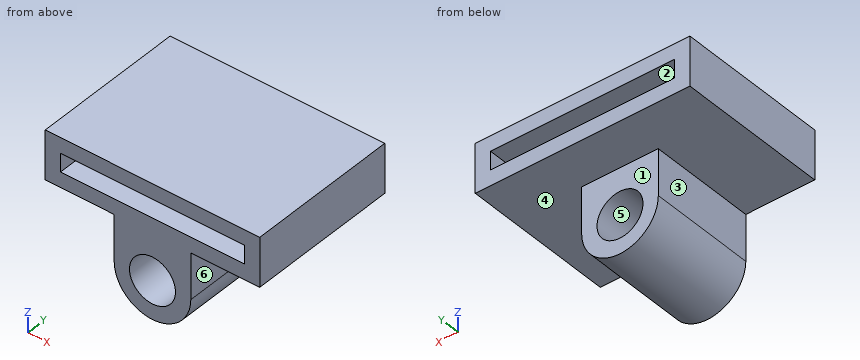
from build123d import *

# Parameters (mm, degrees)
SKETCH1_W                = 14
SKETCH1_H                = 3.2
SKETCH1_W_2              = 12
SKETCH1_H_2              = 1.2
BOSS_EXTRUDE1_DEPTH      = 5
BOSS_EXTRUDE2_DEPTH      = 2
BOSS_EXTRUDE2_DEPTH_BACK = 5
SKETCH1_3_R              = 1.5


with BuildPart() as part:
    # Sketch1 → Boss-Extrude1 (new, symmetric)
    with BuildSketch(Plane(origin=(0, 0, 0), x_dir=(1, 0, 0), z_dir=(0, 1, 0))):
        Rectangle(SKETCH1_W, SKETCH1_H)
        Rectangle(SKETCH1_W_2, SKETCH1_H_2, mode=Mode.SUBTRACT)
    extrude(amount=BOSS_EXTRUDE1_DEPTH, both=True)

    # Sketch1_3 → Boss-Extrude2 (add, two sides: drawn at the far end of the back side and taken through both)
    with BuildSketch(Plane(origin=(0, 0, 0), x_dir=(1, 0, 0), z_dir=(0, 1, 0)).offset(-BOSS_EXTRUDE2_DEPTH_BACK)):
        with BuildLine():
            ThreePointArc((2.5, 4.6), (0, 7.1), (-2.5, 4.6))
            Line((-2.5, 4.6), (-2.5, 1.6))
            Line((-2.5, 1.6), (2.5, 1.6))
            Line((2.5, 1.6), (2.5, 4.6))
        make_face()
        with Locations(Location((0, 4.6, 0), (0, 0, 270))):
            Circle(SKETCH1_3_R, mode=Mode.SUBTRACT)
    extrude(amount=BOSS_EXTRUDE2_DEPTH + BOSS_EXTRUDE2_DEPTH_BACK)


solid = part.part
Design review of the part built by this model. Coordinates are the model's own, in mm. Face numbers are marked on the shaded views. A direction names the side the tool comes from. Give positions to 0.01 mm unless a question says otherwise; leave off trailing zeros. Write each loop counter-clockwise with the first axis right and the second up, starting at its lowest first coordinate (ties: lowest second). Pieces come first, ordered by that corner, then holes. Notation, with made-up numbers: M 35.5,28.25 L 44.5,28.25 A24 cw 44.5,53.25 Z; hole C 36,-3 d7. An arc over 180 degrees is marked long. Return JSON: item names as keys, results as strings. Group by question number.
Item 1: Wall thickness on line 1 along X through (y, z) = (-3, -4.6); line 2 along Z through (x, y) = (4.5, -0.75); line 3 along X through (y, z) = (-4, 0.5): over which ranges is each line inside the solid? List them lowest first.
Item 2: Take a section at D-D (y = -3.75). Give the boundary of the cut face in (x, z).
Item 3: The part is to be moulded in two halves that separate along X. For the marked faces 4, 5 and 6, say which applies: pulls with the +X half, pulls with the -X half, needs draft (parallel to the pull), parting line crosses it, or undercut.
Item 4: Clearance check with flat-ended pins moving along their axes: pin 1 Ø2.5 at (y, z) = (-0.5, -3.5) entering from +X; pin 2 Ø1.5 at (x, z) = (5, -4.5) entering from +Y; pin 3 Ø3 at (x, z) = (4, -0.5) entering from -Y. State where each tip first meets the part, or that it passes through.
Item 5: Take a section at C-C (x = 5). Give the boundary of the cut face in (y, z), plus the area to 3 significant figures.
Item 6: Take a section at A-A (x = 0). Give the boundary of the cut face in (y, z), plus the area to 3 significant figures.
Item 7: Tool access review of the marked faces 1, 2 and 3: name each direction out of +Z, -Z, +X, -X, +Y, -Y from which nothing blocks a thin tool from reaching the whole face with its end or side.
Item 8: Take a section at B-B (y = 4.5). Give the boundary of the cut face in (x, z), plus the area to 3 significant figures.
Return value:
{
 "1": {"line 1": "x = -2.5 to -1.5, 1.5 to 2.5", "line 2": "z = -1.6 to -0.6, 0.6 to 1.6", "line 3": "x = -7 to -6, 6 to 7"},
 "2": {"outline": "M -7,-1.6 L -2.5,-1.6 L -2.5,-4.6 A2.5 ccw 2.5,-4.6 L 2.5,-1.6 L 7,-1.6 L 7,1.6 L -7,1.6 Z; hole M -6,-0.6 L 6,-0.6 L 6,0.6 L -6,0.6 Z; hole C 0,-4.6 d3"},
 "3": {"face 4": "needs draft", "face 5": "undercut", "face 6": "pulls with the +X half"},
 "4": {"pin 1": "stops at x = 2.5", "pin 2": "passes through", "pin 3": "stops at y = -5"},
 "5": {"outline": "M -5,-1.6 L 5,-1.6 L 5,-0.6 L -5,-0.6 Z; M -5,0.6 L 5,0.6 L 5,1.6 L -5,1.6 Z", "area": "20.0 mm2"},
 "6": {"outline": "M -5,-7.1 L 2,-7.1 L 2,-6.1 L -5,-6.1 Z; M -5,-3.1 L 2,-3.1 L 2,-1.6 L 5,-1.6 L 5,-0.6 L -5,-0.6 Z; M -5,0.6 L 5,0.6 L 5,1.6 L -5,1.6 Z", "area": "37.5 mm2"},
 "7": {"face 1": "-Z, +X, -X, +Y", "face 2": "+Y, -Y", "face 3": "-Z, -X, +Y, -Y"},
 "8": {"outline": "M -7,-1.6 L 7,-1.6 L 7,1.6 L -7,1.6 Z; hole M -6,-0.6 L 6,-0.6 L 6,0.6 L -6,0.6 Z", "area": "30.4 mm2"}
}
